Design review of the part built by this model. Coordinates are the model's own, in mm. Face numbers are marked on the shaded views. A direction names the side the tool comes from. Give positions to 0.01 mm unless a question says otherwise; leave off trailing zeros. Write each loop counter-clockwise with the first axis right and the second up, starting at its lowest first coordinate (ties: lowest second). Pieces come first, ordered by that corner, then holes. Notation, with made-up numbers: M 49,-17.5 L 57,-17.5 A4 ccw 57,-10.5 Z; hole C 72.5,-18.5 d5. An arc over 180 degrees is marked long. Write each question's results on one line, items separated by ' | '. Start each with the question number.
from build123d import *

# Parameters (mm, degrees)
F0_R            = 62.480427788
F1_DEPTH        = 63.5
F2_R            = 3.934558481
F3_DEPTH        = 25.4
F3_COPIES_COUNT = 25
F5_DEPTH        = 127


# Not quite as in the source:
# - a pattern or mirror of a feature is missing from the dataset's text; its kind, count and spacing are read off the source's solid


with BuildPart() as f1:
    # F0 (on Front) → F1 (new body, symmetric)
    with BuildSketch(Plane.XZ):
        Circle(F0_R)
    extrude(amount=F1_DEPTH, both=True)

    # F2 (on face) → F3 (join)
    with BuildSketch(Plane.XZ.offset(63.5)):
        with Locations((-38.1652005017, 42.0956611633)):
            Circle(F2_R)
    f3 = extrude(amount=F3_DEPTH)

    # F3_copies: F3 ×25 about axis
    f3_copies_axis = Axis((0, 0, 0), (0, 1, 0))
    for i in range(1, F3_COPIES_COUNT):
        add(f3.rotate(f3_copies_axis, i * 360 / F3_COPIES_COUNT))

    # F4 (on face) → F5 (join)
    with BuildSketch(Plane(origin=(0, 63.5, 0), x_dir=(-1, 0, 0), z_dir=(0, 1, 0))):
        Polygon((24.3383341717, -76.4241799678), (24.3383341717, -57.5451939463), (0, -62.480427788), align=None)
    extrude(amount=-F5_DEPTH)


solid = f1.part
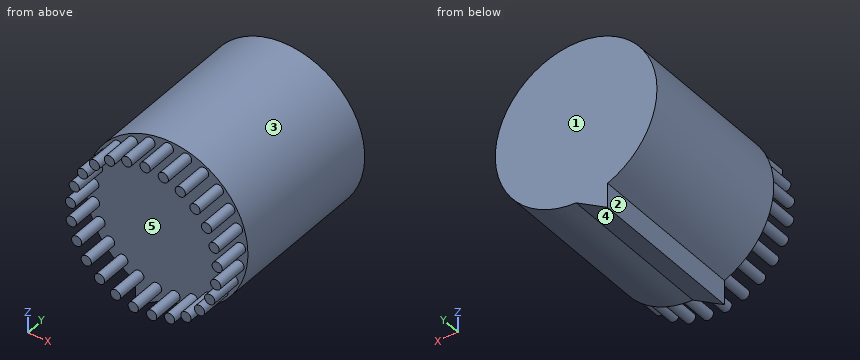
Q1. For the marked faces 1 and 2, list the 3-axis set-ups (+Z, -Z, +X, -X, +Y, -Y) from which the entire face can be reached by the end or side of a thin tool; tool diameter is ignored.
Q2. We need section B-B on z = -67. Write out the cut boundary in (x, y).
Q3. For pin 1 Ø8 at (y, z) = (-0.5, 41.5) entering from -X; pin 2 Ø9.5 at (y, z) = (2, -65.5) entering from -X; pin 3 Ø3 at (y, z) = (18, -26.5) entering from +X, all flat-tipped, find the tip position at first contact; note any pin that passes through.
Q4. Wall thickness on line 1 along Y through (x, z) = (-53, -16); line 2 along X through (y, z) = (-47, -53.5); line 3 along X through (y, z) = (-15.5, -64): over which ranges is each line inside the solid? List them lowest first. Write a range as from..to.
Q5. We need section A-A on y = 3. Write out the cut boundary in (x, z).
Q6. The part is to be moulded in two halves that separate along Z. For the marked faces 3, 4 and 5, say which applies: pulls with the +Z half, pulls with the -Z half, needs draft (parallel to the pull), parting line crosses it, or undercut.
Answer sheet:
1) face 1: +Z, -Z, +X, -X, +Y | face 2: -Z, -X, +Y, -Y
2) outline: M -24.34,-63.5 L -7.89,-63.5 L -7.89,63.5 L -24.34,63.5 Z
3) pin 1: x = -49.98 | pin 2: x = -24.34 | pin 3: x = 57.26
4) line 1: -63.5..63.5 | line 2: -32.27..32.27 | line 3: -24.34..-2.65
5) outline: M -24.34,-76.42 L 0,-62.48 A62.48 ccw long -24.34,-57.55 Z
6) face 3: parting line crosses it | face 4: pulls with the -Z half | face 5: undercut
